Input: part model. Units: mm. Frame: model coordinates. Give positions to 0.01 mm unless a question says otherwise; leave off trailing zeros. Loops run counter-clockwise (first coordinate to the right, second up) from the corner with the lowest first, then second, coordinate; pieces in that order, holes last. Notation, with made-up numbers: M 58,-7.75 L 107,-7.75 A20 cw 107,23.25 Z; hole C 89.5,45.25 d5. An arc over 180 degrees is marked long. Answer as a JSON object with one key per item and string values. Group by question number.
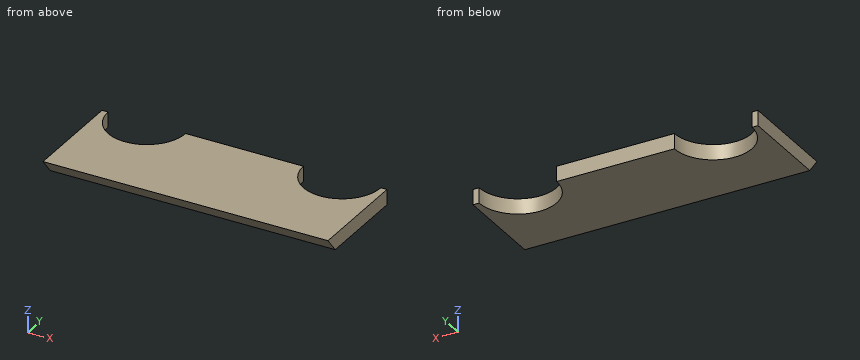
```python
from build123d import *

# Parameters (mm, degrees)
F1_DEPTH = 5
F3_DEPTH = 93.4


with BuildPart() as f1:
    # F0 (on Top) → F1 (new body)
    with BuildSketch(Plane.XY):
        with BuildLine():
            Line((-46.7, 0), (0, 0))
            Line((0, 0), (0, 30))
            Line((0, 30), (-19.3, 30))
            ThreePointArc((-19.3, 30), (-32, 17.3), (-44.7, 30))
            Line((-44.7, 30), (-46.7, 30))
            Line((-46.7, 30), (-46.7, 0))
        make_face()
        with BuildLine():
            Line((0, 30), (0, 0))
            Line((0, 0), (46.7, 0))
            Line((46.7, 0), (46.7, 30))
            Line((46.7, 30), (44.7, 30))
            ThreePointArc((44.7, 30), (32, 17.3), (19.3, 30))
            Line((19.3, 30), (0, 30))
        make_face()
    extrude(amount=F1_DEPTH)

    # F2 (on face) → F3 (join, through all)
    with BuildSketch(Plane(origin=(-46.7, 0, 0), x_dir=(0, -1, 0), z_dir=(-1, 0, 0))):
        Polygon((0, 5), (0, 0), (4.195498, 5), align=None)
    extrude(amount=-F3_DEPTH)


solid = f1.part
```
1. Section B-B (z = 1.15). Output: boundary loops of the cut face in (x, y), then the cut area to 3 significant figures.
2. Section A-A (y = 20). Output: boundary loops of the cut face in (x, z).
3. Section D-D (y = 25.5). Output: boundary loops of the cut face in (x, z).
4. Material intervals for L1, parallel to X at y = 20.5, z = 2.85; L2, parallel to X at y = 23, z = 4.55; L3, parallel to Y at x = -10.5, z = 2.8, sorted ascending.
5. Section C-C (x = 32). Output: boundary loops of the cut face in (y, z), then the cut area to 3 significant figures.
6. First-contact query: P1, Ø6, axis at x = -35.5, y = 1, coming from the -Z side. Flat tip, straight axial feed; report the tip coordinate or a pass-through.
Geometry results:
{
 "1": {"outline": "M -46.7,-0.96 L 46.7,-0.96 L 46.7,30 L 44.7,30 A12.7 cw 19.3,30 L -19.3,30 A12.7 cw -44.7,30 L -46.7,30 Z", "area": "2,390 mm2"},
 "2": {"outline": "M -46.7,0 L -39.83,0 L -39.83,5 L -46.7,5 Z; M -24.17,0 L 24.17,0 L 24.17,5 L -24.17,5 Z; M 39.83,0 L 46.7,0 L 46.7,5 L 39.83,5 Z"},
 "3": {"outline": "M -46.7,0 L -43.88,0 L -43.88,5 L -46.7,5 Z; M -20.12,0 L 20.12,0 L 20.12,5 L -20.12,5 Z; M 43.88,0 L 46.7,0 L 46.7,5 L 43.88,5 Z"},
 "4": {"L1": "-46.7 to -40.43, -23.57 to 23.57, 40.43 to 46.7", "L2": "-46.7 to -42.6, -21.4 to 21.4, 42.6 to 46.7", "L3": "-2.35 to 30"},
 "5": {"outline": "M -4.2,5 L 0,0 L 17.3,0 L 17.3,5 Z", "area": "97.0 mm2"},
 "6": {"P1": "z = 0"}
}
